```python
from build123d import *

# Parameters (mm, degrees)
F1_DEPTH = 76.2
F0_W     = 6.35
F0_H     = 61.992716
F2_DEPTH = 38.1
F3_DEPTH = 25.4


with BuildPart() as f1:
    # F0 (on Front) → F1 (new body)
    with BuildSketch(Plane.XZ):
        Polygon((38.1, -30.996358), (38.1, 30.996358), (31.75, 30.996358), (-44.45, 30.996358), (-44.45, -30.996358), align=None)
    extrude(amount=F1_DEPTH)

    # F0 (on Front) → F2 (join)
    with BuildSketch(Plane.XZ):
        with BuildLine():
            Line((38.1, 30.996358), (44.45, 30.996358))
            Line((44.45, 30.996358), (44.45, 56.396358))
            ThreePointArc((44.45, 56.396358), (47.110789, 62.82007), (53.534501, 65.480859))
            Line((53.534501, 65.480859), (69.985434, 65.480859))
            Line((69.985434, 65.480859), (69.985434, 78.180859))
            Line((69.985434, 78.180859), (53.534501, 78.180859))
            add(Edge.make_bspline(
                [(49.729503, 77.845984), (50.993288, 77.960759), (52.261766, 78.072157), (53.534501, 78.180859)],
                knots=[105.554558, 105.554558, 105.554558, 105.554558, 108.753573, 108.753573, 108.753573, 108.753573], degree=3))
            ThreePointArc((49.729503, 77.845984), (36.839375, 70.390544), (31.75, 56.396358))
            Line((31.75, 56.396358), (31.75, 30.996358))
            Line((31.75, 30.996358), (38.1, 30.996358))
        make_face()
        with Locations((41.275, 0)):
            Rectangle(F0_W, F0_H)
    extrude(amount=F2_DEPTH)

    # F0 (on Front) → F3 (join)
    with BuildSketch(Plane.XZ):
        with BuildLine():
            Line((-44.45, 30.996358), (31.75, 30.996358))
            Line((31.75, 30.996358), (31.75, 56.396358))
            ThreePointArc((31.75, 56.396358), (36.839375, 70.390544), (49.729503, 77.845984))
            add(Edge.make_bspline(
                [(-44.45, 30.996358), (-28.561943, 66.594918), (8.029683, 74.058869), (49.729503, 77.845984)],
                knots=[0, 0, 0, 0, 105.554558, 105.554558, 105.554558, 105.554558], degree=3))
        make_face()
    extrude(amount=F3_DEPTH)

    # F0 (on Front) → F4 (revolve)
    with BuildSketch(Plane.XZ):
        Polygon((69.985434, 78.180859), (69.985434, 65.480859), (69.985434, 57.183055), (109.582732, 57.183055), (109.582732, 79.735152), (69.985434, 79.735152), align=None)
    revolve(axis=Axis((69.985434, 0, 68.459103), (0, 0, -1)))


solid = f1.part
```
Here's how the part is built. I have some questions about the finished solid (model axes, mm). A direction names the side the tool comes from. Give positions to 0.01 mm unless a question says otherwise; leave off trailing zeros. Write each loop counter-clockwise with the first axis right and the second up, starting at its lowest first coordinate (ties: lowest second). Pieces come first, ordered by that corner, then holes. Notation, with made-up numbers: M 24.25,80.5 L 46.25,80.5 A21 ccw 46.25,101.5 Z; hole C -6,75 d3. An arc over 180 degrees is marked long. Put each result on its own line as item: value. Start each with the question number.
Item 1: If we section it at B-B, the plane y = -57: Write out the boundary of the cut face in (x, z).
Item 2: I need wall thicknesses on L1, parallel to X at y = -22.5, z = -19.5; L2, parallel to Z at x = 62, y = -7.5; L3, parallel to X at y = -50, z = 20.5. Which ranges of each line are inside material? Lowest first, please. Write a range as from..to.
Item 3: If we section it at C-C, the plane x = 73.5: Write out the boundary of the cut face in (y, z).
Item 4: Will these pins go through, and if not, where does the flat tip stop? pin 1 (22 mm diameter, centred on x = 51.5, z = 15.5, fed in from -Y); pin 2 (2 mm diameter, centred on y = -56.5, z = 4, fed in from +X); pin 3 (5 mm diameter, centred on y = -33, z = -1, fed in from +X).
Item 5: If we section it at A-A, the plane z = 26.5: Write out the boundary of the cut face in (x, y).
Item 6: On a 3-axis mill with a long thin cutter (end or side, diameter ignored), from which of +Z, -Z, +X, -X, +Y, -Y can I reach the whole of each face in a straight line? I mean faces 1 (the flat face through (6, -25.4, 49)), 2 (the flat face through (-44.45, -38, 0)), 3 (the flat face through (44.45, -19, 12)), 4 (the flat face through (-1, -38, -30.996)), 5 (the flat face through (38.1, -57, 0)). Say none if no direction works.
Values:
1. outline: M -44.45,-31 L 38.1,-31 L 38.1,31 L -44.45,31 Z
2. L1: -44.45..44.45
2. L2: 57.18..79.74
2. L3: -44.45..38.1
3. outline: M -39.44,57.18 L 39.44,57.18 L 39.44,79.74 L -39.44,79.74 Z
4. pin 1: y = -38.1
4. pin 2: x = 38.1
4. pin 3: x = 44.45
5. outline: M -44.45,-76.2 L 38.1,-76.2 L 38.1,-38.1 L 44.45,-38.1 L 44.45,0 L -44.45,0 Z
6. face 1: +Z, -X, -Y
6. face 2: +Z, -Z, -X, +Y, -Y
6. face 3: -Z, +X, +Y, -Y
6. face 4: -Z, +X, -X, +Y, -Y
6. face 5: +Z, -Z, +X, -Y
